Geometry check sheet. Reference: the model listing, model coordinates, mm. A direction names the side the tool comes from. Give positions to 0.01 mm unless a question says otherwise; leave off trailing zeros. Loops run counter-clockwise (first coordinate to the right, second up) from the corner with the lowest first, then second, coordinate; pieces in that order, holes last. Notation, with made-up numbers: (-39, 38) -> (-19, 38) arc R26 cw to (-19, 73) -> close; hole circle Ø11 at (15.25, -10). An arc over 180 degrees is marked (long way). One line per question, with ' | ' between items.
from build123d import *

# Parameters (mm, degrees)
SKETCH_1_R          = 4
EXTRUDE_1_DEPTH     = 40
SKETCH_2_W          = 25
SKETCH_2_H          = 31.038795999
CUT_EXTRUDE_1_DEPTH = 74.745137045
FILLET_3_R          = 2


with BuildPart() as part:
    # 草图1 → 凸台-拉伸1 (new body)
    with BuildSketch(Plane.XY):
        with BuildLine():
            Line((0, 46.226497308), (0, 16.226497308))
            Line((0, 16.226497308), (-8, 16.226497308))
            Line((-8, 16.226497308), (-8, -5.773502692))
            Line((-8, -5.773502692), (19.748711306, -21.794228634))
            ThreePointArc((19.748711306, -21.794228634), (30.019659504, -20.906240432), (32.718489579, -10.956505956))
            Line((32.718489579, -10.956505956), (15.356489888, 37.360423737))
            Line((15.356489888, 37.360423737), (0, 46.226497308))
        make_face()
        Circle(SKETCH_1_R, mode=Mode.SUBTRACT)
        with Locations((24.248711306, -14)):
            Circle(SKETCH_1_R, mode=Mode.SUBTRACT)
    extrude(amount=EXTRUDE_1_DEPTH)

    # 草图2 → 切除-拉伸1 (cut, through all)
    with BuildSketch(Plane.ZY.offset(8)):
        with Locations((20, -9.292900692)):
            Rectangle(SKETCH_2_W, SKETCH_2_H)
    extrude(amount=-CUT_EXTRUDE_1_DEPTH, mode=Mode.SUBTRACT)

    # 圆角3
    fillet_3_edges = [part.edges().sort_by_distance(p)[0] for p in [
        (9.272011192, 6.226497308, 7.5),
        (9.272011192, 6.226497308, 32.5),
    ]]
    fillet(fillet_3_edges, radius=FILLET_3_R)


solid = part.part
Item 1: Sectioned sample at D-D (z = 27). Record the cut outline in (x, y), plus the area to 3 significant figures.
Result:
outline: (-8, 6.23) -> (26.54, 6.23) -> (15.36, 37.36) -> (0, 46.23) -> (0, 16.23) -> (-8, 16.23) -> close | area: 800 mm2
Item 2: Scan lines: probe 1 along Z at (x, y) = (30, -18.5); probe 2 along X at (y, z) = (-14, 3); probe 3 along X at (y, z) = (0, 36). Record each from-to range of solid material in increasing order.
Result:
probe 1: 0 to 7.5, 32.5 to 40 | probe 2: 6.25 to 20.25, 28.25 to 33.25 | probe 3: -8 to -4, 4 to 28.78
Item 3: Depth check by flat-ended pin: pin 1 Ø5 at (x, y) = (0, 0) entering from +Z; pin 2 Ø17 at (x, z) = (6, 19) entering from -Y; pin 3 Ø4 at (x, z) = (24, 10.5) entering from -Y; pin 4 Ø8 at (y, z) = (6, 35.5) entering from +X. Enter the tip coordinate at first touch or a pass-through.
Result:
pin 1: through | pin 2: y = 6.23 | pin 3: y = 5.96 | pin 4: x = 28.06
Item 4: Sectioned sample at A-A (z = 3). Record the cut outline in (x, y), plus the area to 3 significant figures.
Result:
outline: (-8, -5.77) -> (19.75, -21.79) arc R9 ccw to (32.72, -10.96) -> (15.36, 37.36) -> (0, 46.23) -> (0, 16.23) -> (-8, 16.23) -> close; hole circle Ø8 at (0, 0); hole circle Ø8 at (24.25, -14) | area: 1,570 mm2
Item 5: Release check for a two-part mould opening along X. For faces 4 (the face through (0, 31, 20)), 5 (the face through (12, 4, 40)), 6 (the face through (27.944, -15.532, 36.198)) record: pulls with the +X half, pulls with the -X half, needs draft (parallel to the pull), parting line crosses it, or undercut.
Result:
face 4: pulls with the -X half | face 5: needs draft | face 6: undercut
Item 6: Set-up check for faces 1 (the face through (9, 6.226, 20)), 2 (the face through (5.68, -13.67, 3.7)), 3 (the face through (-4, 16.226, 20)): record each of +Z, -Z, +X, -X, +Y, -Y from which the full face is reachable in a straight line by a thin tool's end or side.
Result:
face 1: +X, -X, -Y | face 2: +Z, -Z, -X, -Y | face 3: +Z, -Z, -X, +Y
Item 7: Sectioned sample at C-C (x = 1). Record the cut outline in (y, z).
Result:
outline: (-10.97, 0) -> (-3.87, 0) -> (-3.87, 7.5) -> (-10.97, 7.5) -> close; (-10.97, 32.5) -> (-3.87, 32.5) -> (-3.87, 40) -> (-10.97, 40) -> close; (3.87, 0) -> (45.65, 0) -> (45.65, 40) -> (3.87, 40) -> (3.87, 32.5) -> (4.23, 32.5) arc R2 cw to (6.23, 30.5) -> (6.23, 9.5) arc R2 cw to (4.23, 7.5) -> (3.87, 7.5) -> close
Item 8: Sectioned sample at B-B (y = 0). Record the cut outline in (x, z).
Result:
outline: (-8, 0) -> (-4, 0) -> (-4, 7.5) -> (-8, 7.5) -> close; (-8, 32.5) -> (-4, 32.5) -> (-4, 40) -> (-8, 40) -> close; (4, 0) -> (28.78, 0) -> (28.78, 7.5) -> (4, 7.5) -> close; (4, 32.5) -> (28.78, 32.5) -> (28.78, 40) -> (4, 40) -> close
